Design review of the part built by this model. Coordinates are the model's own, in mm. A direction names the side the tool comes from. Round coordinates to 2 decimals unless told otherwise and drop trailing zeros. Loops run counter-clockwise (first coordinate to the right, second up) from the corner with the lowest first, then second, coordinate; pieces in that order, holes last. Notation, with made-up numbers: (70.5, -25) - (128.5, -25) arc R22 cw to (128.5, -19) - close; hole circle Ø11 at (60.25, -31.5). An arc over 180 degrees is marked (long way). One line per question, with ' | ' between items. Start each with the question number.
Autodesk Inventor part; units mm, degrees
ref_plane "YZ Plane" through (0, 0, 0) normal (1, 0, 0) x (0, 1, 0)
ref_plane "XZ Plane" through (0, 0, 0) normal (0, 1, 0) x (-1, 0, 0)
ref_plane "XY Plane" through (0, 0, 0) normal (0, 0, 1) x (1, 0, 0)
sketch "base" plane through (0, 0, 0) normal (0, 1, 0) x (-1, 0, 0)
  line L0 (35, 50) -> (-35, 50)
  line L1 (-35, 50) -> (-35, -50)
  line L2 (-35, -50) -> (35, -50)
  line L3 (35, -50) -> (35, 50)
  point P0 (0, 0)
  point P1 (0, 0)
  dimension "d0" = 70
  dimension "d1" = 100
  dimension "d2" = 50
  dimension "d3" = 35
  dimension "d4" = 0
  dimension "d5" = 0
extrude "baseBody" add sketch "base" along normal blind 5
fillet "filletBaseBody" radius 8 2 edges at (-35, 2.5, -50) (35, 2.5, 50)
shell "shellBaseBody" thickness 2 removed faces 1 at (11.6667, 5, -16.6667)
sketch "baseBorderCase" plane through (0, 5, 0) normal (0, 1, 0) x (1, 0, 0)
  line L0 (-35, -50) -> (27, -50)
  line L1 (35, -42) -> (35, 50)
  line L2 (35, 50) -> (-27, 50)
  line L3 (-35, 42) -> (-35, -50)
  arc A0 (-27, 50) -> (-35, 42) centre (-27, 42) ccw
  arc A1 (27, -50) -> (35, -42) centre (27, -42) ccw
  line L4 (-34, -49) -> (27, -49)
  arc A2 (27, -49) -> (34, -42) centre (27, -42) ccw
  line L5 (34, -42) -> (34, 49)
  line L6 (34, 49) -> (-27, 49)
  arc A3 (-27, 49) -> (-34, 42) centre (-27, 42) ccw
  line L7 (-34, 42) -> (-34, -49)
  point P0 (0, 0)
  dimension "d10" = 8
  dimension "d11" = 1
extrude "borderCase" add sketch "baseBorderCase" along normal blind 1
sketch "baseFrontHoles" plane through (-35, 0, 50) normal (0, 0, 1) x (1, 0, 0)
  line L0 (2, 2) -> (2, 5)
  line L1 (2, 2) -> (2, 5)
  line L2 (2, 5) -> (4.5, 5)
  line L3 (4.5, 5) -> (4.5, 18.5)
  line L4 (4.5, 18.5) -> (20.5, 18.5)
  line L5 (20.5, 18.5) -> (20.5, 5)
  line L6 (20.5, 5) -> (4.5, 5)
  line L7 (20.5, 5) -> (24.5, 5)
  line L8 (24.5, 5) -> (24.5, 19.5)
  line L9 (24.5, 19.5) -> (38, 19.5)
  line L10 (38, 19.5) -> (38, 5)
  line L11 (38, 5) -> (24.5, 5)
  line L12 (38, 5) -> (43, 5)
  line L13 (43, 5) -> (43, 19.5)
  line L14 (43, 19.5) -> (56.5, 19.5)
  line L15 (56.5, 19.5) -> (56.5, 5)
  line L16 (56.5, 5) -> (43, 5)
  point P0 (35, 0)
  dimension "d14" = 3
  dimension "d15" = 2.5
  dimension "d16" = 13.5
  dimension "d17" = 16
  dimension "d18" = 13.5
  dimension "d19" = 16
  dimension "d20" = 4
  dimension "d21" = 14.5
  dimension "d22" = 13.5
  dimension "d23" = 14.5
  dimension "d24" = 13.5
  dimension "d25" = 5
  dimension "d26" = 14.5
  dimension "d27" = 13.5
  dimension "d28" = 14.5
extrude "frontHoles" cut sketch "baseFrontHoles" against normal up to surface (2 mm away)
sketch "baseLateralHoles" plane through (-35, 0, -42) normal (-1, 0, 0) x (0, 0, 1)
  line L0 (90, 2) -> (90, 5)
  line L1 (90, 2) -> (90, 5)
  line L2 (90, 5) -> (62.5, 5)
  line L3 (62.5, 5) -> (62.5, 11)
  line L4 (62.5, 11) -> (55.5, 11)
  line L5 (55.5, 11) -> (55.5, 5)
  line L6 (55.5, 5) -> (62.5, 5)
  line L7 (55.5, 5) -> (45, 5)
  line L8 (45, 5) -> (45, 11)
  line L9 (45, 11) -> (30, 11)
  line L10 (30, 11) -> (30, 5)
  line L11 (30, 5) -> (45, 5)
  line L12 (30, 5) -> (20, 5)
  line L13 (20, 5) -> (20, 8)
  line L14 (20, 8) -> (12.5, 8)
  line L15 (12.5, 8) -> (12.5, 5)
  line L16 (12.5, 5) -> (20, 5)
  point P0 (42, 0)
  dimension "d31" = 3
  dimension "d32" = 27.5
  dimension "d33" = 6
  dimension "d34" = 7
  dimension "d35" = 10.5
  dimension "d36" = 6
  dimension "d37" = 15
  dimension "d38" = 10
  dimension "d39" = 3
  dimension "d40" = 7.5
extrude "lateralHoles" cut sketch "baseLateralHoles" against normal up to surface (2 mm away)
sketch "baseScrewHolders" plane through (-27, 2, -48) normal (0, 1, 0) x (1, 0, 0)
  line L0 (-1.6495, -96) -> (-1.6495, -72.425)
  circle A0 centre (-1.6495, -72.425) radius 1.25
  line L1 (-1.6495, -72.425) -> (47.3005, -72.425)
  line L2 (47.3005, -72.425) -> (47.3005, -14.925)
  line L3 (47.3005, -14.925) -> (-1.6495, -14.925)
  line L4 (-1.6495, -14.925) -> (-1.6495, -72.425)
  circle A1 centre (47.3005, -72.425) radius 1.25
  circle A2 centre (47.3005, -14.925) radius 1.25
  circle A3 centre (-1.6495, -14.925) radius 1.25
  circle A4 centre (-1.6495, -14.925) radius 3.25
  circle A5 centre (47.3005, -14.925) radius 3.25
  circle A6 centre (47.3005, -72.425) radius 3.25
  circle A7 centre (-1.6495, -72.425) radius 3.25
  point P0 (27, -48)
  point P1 (-6, -96)
  dimension "d44" = 23.575
  dimension "d45" = 2.5
  dimension "d46" = 48.95
  dimension "d47" = 57.5
  dimension "d48" = 2.5
  dimension "d49" = 2.5
  dimension "d50" = 2.5
  dimension "d51" = 6.5
  dimension "d52" = 6.5
  dimension "d53" = 6.5
  dimension "d54" = 6.5
  dimension "d74" = 4.3505
extrude "screwHolders" add sketch "baseScrewHolders" along normal blind 3 contours A7 L4 A0 L0 | L0 A0 L1 A7 | A7 L1 A0 L4 | A4 L3 A3 L4 | L4 A3 L3 A4 | A6 L2 A1 L1 | L1 A1 L2 A6 | A5 L2 A2 L3 | L3 A2 L2 A5
extrude "screwHoles" cut sketch "baseScrewHolders" against normal up to next contours A0 L4 L0 | L0 L1 A0 | L4 A0 L1 | A3 L3 L4 | L4 L3 A3 | A1 L2 L1 | L1 L2 A1 | A2 L2 L3 | L3 L2 A2
chamfer "screwHolderChamfler1" distance 3 angle 10 1 edges at (-31.8995, 5, -33.075) measured on face at (-25.41, 4, -32.8135)
chamfer "screwHolderChamfler2" distance 3 angle 10 1 edges at (17.0505, 5, -33.075) measured on face at (23.54, 4, -32.8135)
chamfer "screwHolderChamfler3" distance 3 angle 10 1 edges at (17.0505, 5, 24.425) measured on face at (23.54, 4, 24.6865)
chamfer "screwHolderChamfler4" distance 3 angle 10 1 edges at (-31.8995, 5, 24.425) measured on face at (-25.41, 4, 24.6865)
chamfer "Chamfer5" distance 2 angle 45 4 edges at (19.0505, 0, 24.425) (-29.8995, 0, 24.425) (-29.8995, 0, -33.075) (19.0505, 0, -33.075)
equation "\"d48\" = d45"
equation "\"d49\" = d48"
equation "\"d50\" = d49"
equation "\"d51\" = d52"
equation "\"d52\" = d53"
equation "\"d53\" = d54"
properties part number "bottom"
1. Machinability: for faces 1 (the face through (31.196, 3.521, 46.289)), 2 (the face through (20, 1.87, -34.42)), which of the approach directions +Z, -Z, +X, -X, +Y, -Y give a long, thin tool a straight path to every point of the face, cutting with its end or side? Answer none if there is none.
2. To check wall thickness, follow line 1 along X through (y, z) = (4.25, -30.5); line 2 along X through (y, z) = (2.5, 22); line 3 along Z through (x, y) = (18, 2.25). State the ranges of each line that lie inside material, in increasing order.
3. Take a section at C-C, the plane x = 0. Give the boundary of the cut face in (y, z).
4. The part is to be moulded in two halves that separate along Z. For faces 3 (the face through (-28.95, 1.87, -34.42)), 4 (the face through (0, 0, 1)), 5 (the face through (-32.594, 3.042, -47.719)), say which applies: pulls with the +Z half, pulls with the -Z half, needs draft (parallel to the pull), parting line crosses it, or undercut.
5. Clearance check with flat-ended pins moving along their axes: P1, Ø0.8, axis at y = 5.5, z = 49.5, coming from the +X side; P2, Ø4, axis at x = -28.65, z = -33.08, coming from the -Y side; P3, Ø5, axis at x = 27, z = 32, coming from the +Y side. State where each tip first meets the part, or that it passes through.
6. Take a section at B-B, the plane z = 14.5. Give the boundary of the cut face in (x, y).
7. Take a section at A-A, the plane y = 3.25. Count the separate pieces of the cut face and the enclosed holes in it, then the cut area to 3 significant figures.
Answer list:
1) face 1: +Y | face 2: -Y
2) line 1: x = -35 to -33, -29.88 to -27.42, 19.07 to 21.53, 33 to 35 | line 2: x = -35 to -33, -30.68 to -26.62, 18.27 to 22.33, 33 to 35 | line 3: z = -50 to -48, -35.31 to -30.84, 22.19 to 26.66, 48 to 50
3) outline: (0, -50) - (6, -50) - (6, -49) - (5, -49) - (5, -48) - (2, -48) - (2, 48) - (5, 48) - (5, 50) - (0, 50) - close
4) face 3: undercut | face 4: needs draft | face 5: pulls with the -Z half
5) P1: stops at x = 30.69 | P2: stops at y = 1.24 | P3: stops at y = 2
6) outline: (-35, 0) - (35, 0) - (35, 6) - (34, 6) - (34, 5) - (33, 5) - (33, 2) - (-33, 2) - (-33, 5) - (-35, 5) - close
7) separate pieces: 5 | enclosed holes: 5 | area: 748 mm²
